Source: CAD feature listing. Evaluate the final solid. Frame: model axes, mm. A direction names the side the tool comes from. Round coordinates to 2 decimals unless told otherwise and drop trailing zeros. Write each loop counter-clockwise with the first axis right and the second up, starting at its lowest first coordinate (ties: lowest second). Pieces come first, ordered by that corner, then holes.
from build123d import *

# Parameters (mm, degrees)
EXTRUDE_1_DEPTH     = 15
FILLET_1_R          = 5
SKETCH_2_R          = 1.6
CUT_EXTRUDE_1_DEPTH = 15
SKETCH_3_R          = 1.6
CUT_EXTRUDE_2_DEPTH = 15


with BuildPart() as part:
    # 草图1 → 凸台-拉伸1 (new body)
    with BuildSketch(Plane(origin=(0, 0, 0), x_dir=(1, 0, 0), z_dir=(0, 1, 0))):
        Polygon((0, 0), (-15, 0), (-15, -15), (-14, -15), (-14, -1), (0, -1), align=None)
    extrude(amount=EXTRUDE_1_DEPTH)

    # 圆角1
    fillet_1_edges = [part.edges().sort_by_distance(p)[0] for p in [
        (-14.5, 15, 15),
        (0, 15, 0.5),
        (-14.5, 0, 15),
        (0, 0, 0.5),
    ]]
    fillet(fillet_1_edges, radius=FILLET_1_R)

    # 草图2 → 切除-拉伸1 (cut)
    with BuildSketch(Plane(origin=(0, 0, 0), x_dir=(-1, 0, 0), z_dir=(0, 0, -1))):
        with Locations((7, 11)):
            Circle(SKETCH_2_R)
        with Locations((7, 4)):
            Circle(SKETCH_2_R)
    extrude(amount=-CUT_EXTRUDE_1_DEPTH, mode=Mode.SUBTRACT)

    # 草图3 → 切除-拉伸2 (cut)
    with BuildSketch(Plane.ZY.offset(15)):
        with Locations((8, 11)):
            Circle(SKETCH_3_R)
        with Locations((8, 4)):
            Circle(SKETCH_3_R)
    extrude(amount=-CUT_EXTRUDE_2_DEPTH, mode=Mode.SUBTRACT)


solid = part.part
1) Pull-direction query (Y, two-part tool) for faces 3 (the face through (-7, 7, 0)), 4 (the face through (-5.4, 11.07, 0.49)), 5 (the face through (-5.73, 3.03, 0.49)), 6 (the face through (-1.43, 1.5, 0.49)); classes: released by +Y, released by -Y, zero draft, split by the parting line, or undercut.
Taken from the geometry:
face 3: zero draft
face 4: undercut
face 5: undercut
face 6: released by -Y
2) Contact query for flat-ended pins moving along their axis: P1, Ø4, axis at y = 4.5, z = 6, coming from the +X side; P2, Ø1.5, axis at x = -4, y = 5, coming from the +Z side. Output: stop coordinate, or through.
Taken from the geometry:
P1: stops at x = -14
P2: stops at z = 1
3) Material intervals for line 1 (Y direction, x = -7, z = 0.3); line 2 (X direction, y = 8.25, z = 11.5); line 3 (Z direction, x = -3.5, y = 13.25), sorted ascending.
Taken from the geometry:
line 1: y = 0 to 2.4, 5.6 to 9.4, 12.6 to 15
line 2: x = -15 to -14
line 3: z = 0 to 1
4) Section query A-A on x = -7. Return the cut outline in (y, z).
Taken from the geometry:
outline: (0, 0) - (2.4, 0) - (2.4, 1) - (0, 1) - close; (5.6, 0) - (9.4, 0) - (9.4, 1) - (5.6, 1) - close; (12.6, 0) - (15, 0) - (15, 1) - (12.6, 1) - close
5) Section query D-D on y = 13.5. Return the cut outline in (x, z).
Taken from the geometry:
outline: (-15, 0) - (-1.43, 0) - (-1.43, 1) - (-14, 1) - (-14, 13.57) - (-15, 13.57) - close
6) Section query C-C on y = 10.25. Return the cut outline in (x, z).
Taken from the geometry:
outline: (-15, 0) - (-8.41, 0) - (-8.41, 1) - (-14, 1) - (-14, 6.59) - (-15, 6.59) - close; (-15, 9.41) - (-14, 9.41) - (-14, 14.99) - (-15, 14.99) - close; (-5.59, 0) - (-0.01, 0) - (-0.01, 1) - (-5.59, 1) - close
7) Section query B-B on z = 8. Return the cut outline in (x, y), then the cut area to 3 significant figures.
Taken from the geometry:
outline: (-15, 0) - (-14, 0) - (-14, 2.4) - (-15, 2.4) - close; (-15, 5.6) - (-14, 5.6) - (-14, 9.4) - (-15, 9.4) - close; (-15, 12.6) - (-14, 12.6) - (-14, 15) - (-15, 15) - close
area: 8.60 mm2
8) Reachability of faces 1 (the face through (-14.51, 11.07, 6.4)), 2 (the face through (-7, 7, 1)) from +Z, -Z, +X, -X, +Y, -Y: full face, straight path, thin tool, end or side. Return the list, or none.
Taken from the geometry:
face 1: +X, -X
face 2: +Z, +X, +Y, -Y
